from build123d import *

# Parameters (mm, degrees)
SKETCH1_R           = 6.35
SKETCH1_R_2         = 9.5
BOSS_EXTRUDE1_DEPTH = 13.75
SKETCH3_R           = 6.35
CUT_EXTRUDE1_DEPTH  = 6
SKETCH4_W           = 38
SKETCH4_H           = 13.5
CUT_EXTRUDE2_DEPTH  = 83.330365488
CUT_EXTRUDE3_DEPTH  = 5
CUT_EXTRUDE3_DRAFT  = -5


with BuildPart() as part:
    # Sketch1 → Boss-Extrude1 (new body, symmetric)
    with BuildSketch(Plane.XY):
        with BuildLine():
            Line((0, 0), (0, 14.5))
            Line((0, 14.5), (-22, 14.5))
            ThreePointArc((-22, 14.5), (-28.5, 21), (-22, 27.5))
            Line((-22, 27.5), (0, 27.5))
            Line((0, 27.5), (0, 36))
            ThreePointArc((0, 36), (-33.793604177, 47.289264213), (-57.021595035, 74.306214643))
            ThreePointArc((-57.021595035, 74.306214643), (-73.547441909, 81.786196516), (-83.58403216, 66.675915252))
            Line((-83.58403216, 66.675915252), (-77.852848425, 18.518324646))
            ThreePointArc((-77.852848425, 18.518324646), (-70.944260783, 5.297847561), (-57, 0))
            Line((-57, 0), (0, 0))
        make_face()
        with Locations((-69.68213321, 68.330365488)):
            Circle(SKETCH1_R, mode=Mode.SUBTRACT)
        with Locations((-57, 21)):
            Circle(SKETCH1_R_2, mode=Mode.SUBTRACT)
    extrude(amount=BOSS_EXTRUDE1_DEPTH, both=True)

    # Sketch3 → Cut-Extrude1 (cut)
    with BuildSketch(Plane.XY.offset(13.75)):
        with BuildLine():
            ThreePointArc((-57.021595035, 74.306214643), (-73.547441909, 81.786196516), (-83.58403216, 66.675915252))
            Line((-83.58403216, 66.675915252), (-82.066046583, 53.920692017))
            ThreePointArc((-82.066046583, 53.920692017), (-66.211511297, 49.650034026), (-52.948932679, 59.330365488))
            Line((-52.948932679, 59.330365488), (-47.326454774, 59.330365488))
            ThreePointArc((-47.326454774, 59.330365488), (-52.674708251, 66.494155172), (-57.021595035, 74.306214643))
        make_face()
        with Locations((-69.68213321, 68.330365488)):
            Circle(SKETCH3_R, mode=Mode.SUBTRACT)
    cut_extrude1 = extrude(amount=-CUT_EXTRUDE1_DEPTH, mode=Mode.SUBTRACT)

    # Mirror1: Cut-Extrude1 across plane
    add(cut_extrude1.mirror(Plane.XY), mode=Mode.SUBTRACT)

    # Sketch4 → Cut-Extrude2 (cut, through all)
    with BuildSketch(Plane.XZ):
        with Locations((-19, 0)):
            Rectangle(SKETCH4_W, SKETCH4_H)
    extrude(amount=-CUT_EXTRUDE2_DEPTH, mode=Mode.SUBTRACT)


with BuildPart() as cut_extrude3_tool:
    # Sketch5 → Cut-Extrude3 (with draft: the straight prism first)
    with BuildSketch(Plane.XY.offset(13.75)):
        with BuildLine():
            ThreePointArc((-51.79358939, 57.330365488), (-64.185224634, 48.062558599), (-79.561455233, 49.799337552))
            Line((-79.561455233, 49.799337552), (-75.866862861, 18.75467468))
            ThreePointArc((-75.866862861, 18.75467468), (-69.616235946, 6.79329065), (-57, 2))
            Line((-57, 2), (-2, 2))
            Line((-2, 2), (-2, 12.5))
            Line((-2, 12.5), (-22, 12.5))
            ThreePointArc((-22, 12.5), (-30.5, 21), (-22, 29.5))
            Line((-22, 29.5), (-2, 29.5))
            Line((-2, 29.5), (-2, 34.12995492))
            ThreePointArc((-2, 34.12995492), (-27.376011233, 41.232719036), (-48.238824631, 57.330365488))
            Line((-48.238824631, 57.330365488), (-51.79358939, 57.330365488))
        make_face()
    extrude(amount=-CUT_EXTRUDE3_DEPTH)
    # Cut-Extrude3: the draft: its side faces are tilted about the plane it starts from
    cut_extrude3_sides = [cut_extrude3_tool.faces().sort_by_distance(p)[0] for p in [
        (-50.01620701, 57.330365488, 11.25),
        (-64.185224634, 48.062558599, 11.25),
        (-77.714159047, 34.277006116, 11.25),
        (-69.616235946, 6.79329065, 11.25),
        (-29.5, 2, 11.25),
        (-2, 7.25, 11.25),
        (-12, 12.5, 11.25),
        (-30.5, 21, 11.25),
        (-12, 29.5, 11.25),
        (-2, 31.81497746, 11.25),
        (-27.376011233, 41.232719036, 11.25),
    ]]
    draft(cut_extrude3_sides, Plane.XY.offset(13.75), CUT_EXTRUDE3_DRAFT)


with BuildPart() as part_1:
    add(part.part)

    # Cut-Extrude3: cut by cut_extrude3_tool
    add(cut_extrude3_tool.part, mode=Mode.SUBTRACT)


solid = part_1.part
Check sheet for the modelled part. Datum: model origin and axes. Units: mm. A direction names the side the tool comes from. Round coordinates to 2 decimals unless told otherwise and drop trailing zeros. Write each loop counter-clockwise with the first axis right and the second up, starting at its lowest first coordinate (ties: lowest second). Pieces come first, ordered by that corner, then holes. Notation, with made-up numbers: (-17, 27) -> (32, 27) arc R12 cw to (32, 47) -> close; hole circle Ø9 at (-8.75, 28.25). An arc over 180 degrees is marked (long way). Answer as CSV lines item,"result". Start each with the question number.
1) Material ranges on line 1 (Z direction, x = -27.5, y = 8); line 2 (Y direction, x = -57, z = 2.25); line 3 (X direction, y = 9.5, z = 12), recorded low to high. Write a range as from..to.
2) Section check B-B on y = 21. Enter the section's corners in (x, z).
3) Tool access check on faces 5 (the flat face through (-42, 0, 0)), 6 (the conical face through (-30.714, 20.808, 11.285)), 7 (the flat face through (-29, 25, 13.75)), 8 (the flat face through (-11, 27.5, 10)), 9 (the flat face through (-38, 25, 0)). Record the directions out of +Z, -Z, +X, -X, +Y, -Y that give a thin tool (end or side, any length) a straight path to the whole face; none if there is none.
4) Go/stop test with flat-tipped pins: P1, Ø24.5, axis at x = -57, y = 21, coming from the +Z side; P2, Ø1.5, axis at y = 41.5, z = -9, coming from the +X side; P3, Ø1, axis at y = 56, z = 2.5, coming from the +X side. Record where each tip stops, or that it passes through.
5) Release check for a two-part mould opening along X. For faces 1 (the cylindrical face through (-71.1, 5.44, 0.19)), 2 (the flat face through (-23, 14, 6.75)), 3 (the cylindrical face through (-76.026, 68.61, -0.109)), 4 (the cylindrical face through (-28.5, 20.9, -10.2)) record: pulls with the +X half, pulls with the -X half, needs draft (parallel to the pull), parting line crosses it, or undercut.
6) Section check A-A on y = 65.5. Enter the section's corners in (x, z), and give its area (3 significant figures).
Found:
1,line 1,"z = -13.75..-6.75, 6.75..8.75"
1,line 2,"y = 0..11.5, 30.5..74.26"
1,line 3,"x = -74.57..-71.93, -2.15..0"
2,outline,"(-78.15, -13.75) -> (-66.5, -13.75) -> (-66.5, 8.75) -> (-75.69, 8.75) -> (-76.13, 13.75) -> (-78.15, 13.75) -> close; (-47.5, -13.75) -> (-28.5, -13.75) -> (-28.5, -6.75) -> (-38, -6.75) -> (-38, 6.75) -> (-28.5, 6.75) -> (-28.5, 13.75) -> (-30.5, 13.75) -> (-30.94, 8.75) -> (-47.5, 8.75) -> close"
3,face 5,"+Z, -Z, +X, -X, -Y"
3,face 6,"+Z"
3,face 7,"+Z, +X, -X, +Y, -Y"
3,face 8,"+Z, -Z, +X"
3,face 9,"+X, +Y, -Y"
4,P1,"stops at z = 8.75"
4,P2,"stops at x = -21.45"
4,P3,"stops at x = -43.78"
5,face 1,"pulls with the -X half"
5,face 2,"needs draft"
5,face 3,"undercut"
5,face 4,"pulls with the +X half"
6,outline,"(-83.44, -7.75) -> (-75.37, -7.75) -> (-75.37, 7.75) -> (-83.44, 7.75) -> close; (-64, -7.75) -> (-52.02, -7.75) -> (-52.02, 7.75) -> (-64, 7.75) -> close"
6,area,"311 mm^2"
